Autodesk Fusion 360 part; units mm, degrees
ref_plane "WorkPlane1" through (0, 0, 123.8) normal (0, 0, 1) x (1, 0, 0)
sketch "Sketch1" plane through (0, 0, 123.8) normal (0, 0, 1) x (1, 0, 0)
  circle A0 centre (-85.5, 170) radius 1.4 construction
  line L0 (-81.5, 4) -> (-81.5, 166) construction
  line L1 (-81.5, 166) -> (-81.5, 167) construction
  line L2 (-81.5, 167) -> (-77.5, 167) construction
  line L3 (-77.5, 167) -> (-77.5, 174) construction
  line L4 (-77.5, 174) -> (-81.5, 174) construction
  line L5 (-81.5, 174) -> (-86.5, 174) construction
  line L6 (-87.2574, 174) -> (-87.5, 174) construction
  line L7 (-87.5, 174) -> (-89.5, 172) construction
  line L8 (-89.5, 172) -> (-89.5, 0) construction
  line L9 (-89.5, 0) -> (-81.5, 0) construction
  line L10 (-81.5, 0) -> (-81.5, 4) construction
  circle A1 centre (85.5, 170) radius 1.4 construction
  line L11 (89.5, 0) -> (89.5, 172) construction
  line L12 (89.5, 172) -> (87.5, 174) construction
  line L13 (87.5, 174) -> (86.5, 174) construction
  line L14 (86.5, 174) -> (86.5, 177) construction
  line L15 (86.5, 177) -> (86.45, 177) construction
  line L16 (86.45, 177) -> (86.45, 174) construction
  line L17 (86.45, 174) -> (81.5, 174) construction
  line L18 (81.5, 174) -> (77.5, 174) construction
  line L19 (77.5, 174) -> (77.5, 167) construction
  line L20 (77.5, 167) -> (81.5, 167) construction
  line L21 (81.5, 167) -> (81.5, 0) construction
  line L22 (81.5, 0) -> (89.5, 0) construction
  line L23 (81.5, 0) -> (81.5, -37.7937) construction
  line L24 (81.5, -37.7937) -> (87.5, -37.7937) construction
  line L25 (87.5, -37.7937) -> (89.5, -35.7937) construction
  line L26 (89.5, -35.7937) -> (89.5, -5) construction
  line L27 (89.5, -5) -> (89.5, 0) construction
  line L28 (89.5, 0) -> (81.5, 0) construction
  line L29 (-89.5, 0) -> (-89.5, -35.7937) construction
  line L30 (-89.5, -35.7937) -> (-87.5, -37.7937) construction
  line L31 (-87.5, -37.7937) -> (-81.5, -37.7937) construction
  line L32 (-81.5, -37.7937) -> (-81.5, -5) construction
  line L33 (-81.5, -5) -> (-81.5, 0) construction
  line L34 (-81.5, 0) -> (-89.5, 0) construction
  line L35 (87.5, -37.7937) -> (-87.5, -37.7937) construction
  line L36 (-77.3, 174) -> (77.3, 174) construction
  line L37 (-77.5, 174) -> (77.5, 174)
  line L38 (77.5, 174) -> (87.5, 174)
  line L39 (87.5, 174) -> (89.5, 172)
  line L40 (89.5, 172) -> (89.5, -35.7937)
  line L41 (89.5, -35.7937) -> (87.5, -37.7937)
  line L42 (-87.5, -37.7937) -> (87.5, -37.7937)
  line L43 (-87.5, -37.7937) -> (-89.5, -35.7937)
  line L44 (-89.5, -35.7937) -> (-89.5, 172)
  line L45 (-89.5, 172) -> (-87.5, 174)
  line L46 (-87.5, 174) -> (-77.3, 174)
  circle A2 centre (-85.5, 170) radius 1.8
  circle A3 centre (-85.5, 102) radius 1.8
  circle A4 centre (-85.5, 34) radius 1.8
  circle A5 centre (-85.5, -34) radius 1.8
  circle A6 centre (85.5, -34) radius 1.8
  circle A7 centre (85.5, 34) radius 1.8
  circle A8 centre (85.5, 102) radius 1.8
  circle A9 centre (85.5, 170) radius 1.8
  line L47 (-86.5, 174) -> (-87.2574, 174)
  circle A10 centre (85.5, -34) radius 1.4 construction
  circle A11 centre (-85.5, -34) radius 1.4 construction
  circle A12 centre (-85.5, 34) radius 1.4 construction
  circle A13 centre (-85.5, 102) radius 1.4 construction
  circle A14 centre (85.5, 102) radius 1.4 construction
  circle A15 centre (85.5, 34) radius 1.4 construction
  line L48 (-89.5, 68.1031) -> (89.5, 68.1031) construction
  line L49 (-89.5, 67.9531) -> (89.5, 67.9531)
  line L50 (-77.5, 173.8) -> (-77.3, 173.8)
  line L51 (-77.3, 173.8) -> (77.5, 173.8)
  line L52 (77.5, 173.8) -> (87.4172, 173.8)
  line L53 (87.4172, 173.8) -> (89.3, 171.9172)
  line L54 (89.3, 171.9172) -> (89.3, -35.7109)
  line L55 (89.3, -35.7109) -> (87.4172, -37.5937)
  line L56 (-87.4172, -37.5937) -> (87.4172, -37.5937)
  line L57 (-87.4172, -37.5937) -> (-89.3, -35.7109)
  line L58 (-89.3, -35.7109) -> (-89.3, 171.9172)
  line L59 (-89.3, 171.9172) -> (-87.4172, 173.8)
  line L60 (-87.4172, 173.8) -> (-77.3, 173.8)
  dimension "d2" = 0.2
  dimension "d4" = 3.6
  dimension "d5" = 3.6
  dimension "d6" = 3.6
  dimension "d7" = 3.6
  dimension "d8" = 3.6
  dimension "d9" = 3.6
  dimension "d10" = 3.6
  dimension "d11" = 3.6
  dimension "d14" = 0.15
extrude "Extrude1" add sketch "Sketch1" along normal blind 3 contours L49 L54 L55 L56 L57 L58
sketch "Sketch2" plane through (0, 0, 126.8) normal (0, 0, 1) x (-1, 0, 0)
  circle A0 centre (85.5, 34) radius 1.8
  circle A1 centre (-85.5, 34) radius 1.8
  circle A2 centre (-85.5, -34) radius 1.8
  circle A3 centre (85.5, -34) radius 1.8
  line L0 (87.4172, 37.5937) -> (-87.4172, 37.5937)
  line L1 (-87.4172, 37.5937) -> (-89.3, 35.7109)
  line L2 (-89.3, 35.7109) -> (-89.3, -67.9531)
  line L3 (-89.3, -67.9531) -> (89.3, -67.9531)
  line L4 (89.3, -67.9531) -> (89.3, 35.7109)
  line L5 (89.3, 35.7109) -> (87.4172, 37.5937)
  line L6 (0, -67.9531) -> (0, 37.5937) construction
  line L7 (0, -67.9531) -> (0, -32.9531) construction
  line L8 (0, -32.9531) -> (-63.5, -32.9531) construction
  circle A4 centre (-63.5, -32.9531) radius 1.8
  circle A5 centre (63.5, -32.9531) radius 1.8
  dimension "d15" = 35
  dimension "d16" = 63.5
  dimension "d17" = 3.6
extrude "Extrude2" cut sketch "Sketch2" against normal blind 3 contours A4 | A5
sketch "Sketch3" plane through (0, 0, 126.8) normal (0, 0, 1) x (-1, 0, 0)
  circle A0 centre (-63.5, -32.9531) radius 1.8
  circle A1 centre (63.5, -32.9531) radius 1.8
  circle A2 centre (85.5, 34) radius 1.8
  circle A3 centre (-85.5, 34) radius 1.8
  circle A4 centre (-85.5, -34) radius 1.8
  circle A5 centre (85.5, -34) radius 1.8
  line L0 (87.4172, 37.5937) -> (-87.4172, 37.5937)
  line L1 (-87.4172, 37.5937) -> (-89.3, 35.7109)
  line L2 (-89.3, 35.7109) -> (-89.3, -67.9531)
  line L3 (-89.3, -67.9531) -> (89.3, -67.9531)
  line L4 (89.3, -67.9531) -> (89.3, 35.7109)
  line L5 (89.3, 35.7109) -> (87.4172, 37.5937)
  line L6 (0, -67.9531) -> (0, -57.9531) construction
  line L7 (0, -57.9531) -> (0, 27.0469) construction
  line L8 (0, -15.4531) -> (-55, -15.4531) construction
  line L9 (0, -15.4531) -> (55, -15.4531) construction
  line L10 (1.5, -13.9531) -> (55, -13.9531)
  line L11 (-1.5, -13.9531) -> (-55, -13.9531)
  line L12 (1.5, -16.9531) -> (55, -16.9531)
  line L13 (-1.5, -16.9531) -> (-55, -16.9531)
  line L14 (-55, -16.9531) -> (-55, -13.9531)
  line L15 (55, -16.9531) -> (55, -13.9531)
  line L16 (-1.5, -57.9531) -> (1.5, -57.9531)
  line L17 (1.5, 27.0469) -> (-1.5, 27.0469)
  line L18 (1.5, -57.9531) -> (1.5, -16.9531)
  line L19 (1.5, -13.9531) -> (1.5, 27.0469)
  line L20 (-1.5, -57.9531) -> (-1.5, -16.9531)
  line L21 (-1.5, -13.9531) -> (-1.5, 27.0469)
  dimension "d20" = 10
  dimension "d21" = 85
  dimension "d22" = 55
  dimension "d23" = 55
extrude "Extrude3" add sketch "Sketch3" along normal blind 2 contours L10 L11 L12 L13 L14 L15 L16 L17 L18 L19 L20 L21
fillet "Fillet1" radius 1 12 edges at (-28.25, 13.9531, 126.8) (-1.5, -6.5469, 126.8) (-55, 15.4531, 126.8) (0, -27.0469, 126.8) (1.5, -6.5469, 126.8) (28.25, 13.9531, 126.8) (1.5, 37.4531, 126.8) (55, 15.4531, 126.8) (28.25, 16.9531, 126.8) (0, 57.9531, 126.8) (-28.25, 16.9531, 126.8) (-1.5, 37.4531, 126.8) 1 faces at (19.3333, 15.9531, 128.8)
equation "large_m3 = 3.6 mm"
equation "d4 = large_m3"
equation "d5 = d4"
equation "d6 = d4"
equation "d7 = d4"
equation "d8 = d4"
equation "d9 = d4"
equation "d10 = d4"
equation "d11 = d4"
equation "d16 = ( 127 / 2 ) * 1 mm"
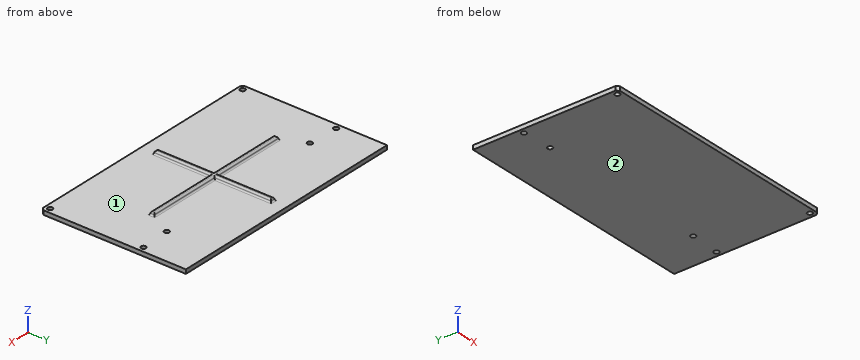
Work out the finished part from the listing and answer in its coordinate system (mm). Face numbers are marked on the shaded views. A direction names the side the tool comes from. Give positions to 0.01 mm unless a question says otherwise; leave off trailing zeros. Order: outer loops, then holes, each group sorted by start corner. A loop starts at its lowest first (then second) coordinate and runs counter-clockwise, first axis right, second up. Notation, with made-up numbers: M 16.5,-19 L 56.5,-19 A21 cw 56.5,-4 Z; hole C 32,-13 d9. An arc over 180 degrees is marked long. Return JSON: item names as keys, results as strings.
Q1. Find the intervals of material crossed by line 1 along Y through (x, z) = (-85.5, 125.9); line 2 along Z through (x, y) = (-59, 27); line 3 along Y through (x, z) = (-63.5, 125.55), in increasing order. Write a range as [from, to].
Answer below:
{"line 1": "y = [-37.59, -35.8], [-32.2, 32.2], [35.8, 67.95]", "line 2": "z = [123.8, 126.8]", "line 3": "y = [-37.59, 31.15], [34.75, 67.95]"}
Q2. Each of these flat-tipped pins is pushed along its axis until it touches: pin 1 (6 mm diameter, centred on x = -85.5, y = -34, fed in from +Z); pin 2 (2 mm diameter, centred on y = -12.5, z = 127, fed in from +X). Where does it stop, or does it pass through?
Answer below:
{"pin 1": "stops at z = 126.8", "pin 2": "stops at x = 89.3"}
Q3. Find section B-B, the plane y = -34. Write down the section's boundary in (x, z).
Answer below:
{"outline": "M -89.3,123.8 L -87.3,123.8 L -87.3,126.8 L -89.3,126.8 Z; M -83.7,123.8 L 83.7,123.8 L 83.7,126.8 L -83.7,126.8 Z; M 87.3,123.8 L 89.3,123.8 L 89.3,126.8 L 87.3,126.8 Z"}
Q4. Which of the six approach directions +Z, -Z, +X, -X, +Y, -Y give full straight-line access (tool end or side, diameter ignored) to the marked faces 1 and 2?
Answer below:
{"face 1": "+Z", "face 2": "-Z, +X, -X, +Y, -Y"}
Q5. Find section A-A, the plane x = -63.5. Write down the section's boundary in (y, z), and give its area (3 significant figures).
Answer below:
{"outline": "M -37.59,123.8 L 31.15,123.8 L 31.15,126.8 L -37.59,126.8 Z; M 34.75,123.8 L 67.95,123.8 L 67.95,126.8 L 34.75,126.8 Z", "area": "306 mm^2"}
Q6. Find section C-C, the plane x = -85.5. Write down the section's boundary in (y, z).
Answer below:
{"outline": "M -37.59,123.8 L -35.8,123.8 L -35.8,126.8 L -37.59,126.8 Z; M -32.2,123.8 L 32.2,123.8 L 32.2,126.8 L -32.2,126.8 Z; M 35.8,123.8 L 67.95,123.8 L 67.95,126.8 L 35.8,126.8 Z"}
